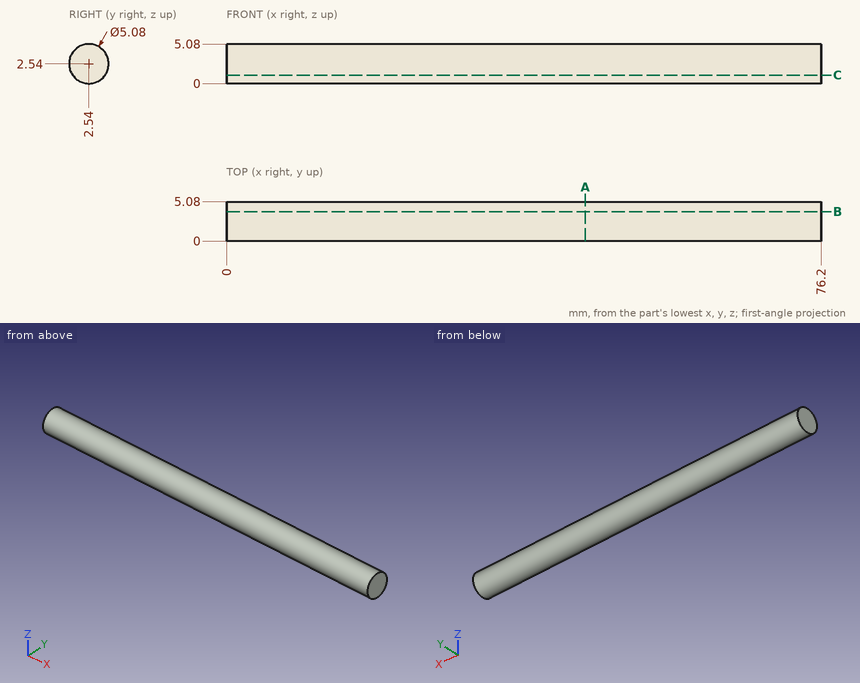
The drawing under review shows one solid part. Ordinate dimensions are in mm from its lowest x, y, z. Coordinates: 2 decimals unless noted, no trailing zeros. Write each loop counter-clockwise with the first axis right and the second up, starting at its lowest first coordinate (ties: lowest second). Pieces come first, ordered by that corner, then holes. Notation, with made-up numbers: (-3, -31.5) -> (22, -31.5) arc R31 ccw to (22, 5.5) -> close; hole circle Ø3 at (-18.5, 34). An arc over 180 degrees is marked (long way). One line per item, written item: value. Start each with the question number.
Q1. Add section A-A, the plane x = 46. Give the boundary of the cut face in (y, z), then the cut area to 3 significant figures.
Q2. Add section B-B, the plane y = 3.8. Give the boundary of the cut face in (x, z), then the cut area to 3 significant figures.
Q3. Add section C-C, the plane z = 1.1. Give the boundary of the cut face in (x, y).
Q4. Clearance check with flat-ended pins moving along their axes: P1, Ø1.5, axis at x = 65, y = 4, coming from the +Z side; P2, Ø1, axis at x = 26, y = 1.5, coming from the -Z side; P3, Ø1.5, axis at x = 47.5, y = 2, coming from the +Z side. State where each tip first meets the part, or that it passes through.
Q5. To check wall thickness, follow probe 1 along Z at (x, y) = (29, 2.4); probe 2 along Y at (x, z) = (51.5, 2.7); probe 3 along Y at (x, z) = (61.5, 3.95). State the ranges of each line that lie inside material, in increasing order.
Response:
1. outline: circle Ø5.08 at (2.54, 2.54)
1. area: 20.3 mm²
2. outline: (0, 0.33) -> (76.2, 0.33) -> (76.2, 4.75) -> (0, 4.75) -> close
2. area: 336 mm²
3. outline: (0, 0.45) -> (76.2, 0.45) -> (76.2, 4.63) -> (0, 4.63) -> close
4. P1: z = 4.98
4. P2: z = 0.06
4. P3: z = 5.08
5. probe 1: 0 to 5.08
5. probe 2: 0.01 to 5.07
5. probe 3: 0.43 to 4.65
